from build123d import *

# Parameters (mm, degrees)
SKETCH1_W           = 21.3
SKETCH1_H           = 15.3
BOSS_EXTRUDE1_DEPTH = 1.7
BOSS_EXTRUDE2_START = 1.7
SKETCH1_3_W         = 3
SKETCH1_3_H         = 2.5
BOSS_EXTRUDE2_DEPTH = 0.9
SKETCH1_4_R         = 0.5
SKETCH1_4_R_2       = 1.5
CUT_EXTRUDE1_DEPTH  = 14.368058947


with BuildPart() as part:
    # Sketch1 → Boss-Extrude1 (new body)
    with BuildSketch(Plane.XY):
        Rectangle(SKETCH1_W, SKETCH1_H)
    extrude(amount=BOSS_EXTRUDE1_DEPTH)

    # Sketch1<3> → Boss-Extrude2 (add)
    with BuildSketch(Plane.XY.offset(BOSS_EXTRUDE2_START)):
        with Locations((0, 2.4)):
            Rectangle(SKETCH1_3_W, SKETCH1_3_H)
    extrude(amount=BOSS_EXTRUDE2_DEPTH)

    # Sketch1<4> → Cut-Extrude1 (cut, through all)
    with BuildSketch(Plane.XY):
        with Locations(Location((3.857142857, -6.4, 0), (0, 0, 180))):
            Circle(SKETCH1_4_R)
        with Locations(Location((-8.65, 5.65, 0), (0, 0, 180))):
            Circle(SKETCH1_4_R_2)
        with Locations(Location((8.65, 5.65, 0), (0, 0, 180))):
            Circle(SKETCH1_4_R_2)
        with Locations(Location((-9, -6.4, 0), (0, 0, 180))):
            Circle(SKETCH1_4_R)
        with Locations(Location((-6.428571429, -6.4, 0), (0, 0, 180))):
            Circle(SKETCH1_4_R)
        with Locations(Location((-3.857142857, -6.4, 0), (0, 0, 180))):
            Circle(SKETCH1_4_R)
        with Locations(Location((-1.285714286, -6.4, 0), (0, 0, 180))):
            Circle(SKETCH1_4_R)
        with Locations(Location((1.285714286, -6.4, 0), (0, 0, 180))):
            Circle(SKETCH1_4_R)
        with Locations(Location((6.428571429, -6.4, 0), (0, 0, 180))):
            Circle(SKETCH1_4_R)
        with Locations(Location((9, -6.4, 0), (0, 0, 180))):
            Circle(SKETCH1_4_R)
    extrude(amount=CUT_EXTRUDE1_DEPTH, mode=Mode.SUBTRACT)


solid = part.part
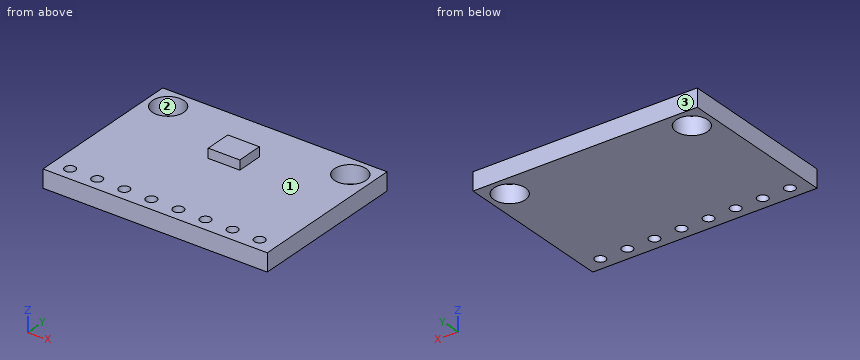
The listing builds one solid part. Answer for the finished solid, in the listing's coordinates (mm). Face numbers are marked on the shaded views. Give positions to 0.01 mm unless a question says otherwise; leave off trailing zeros. Write each loop counter-clockwise with the first axis right and the second up, starting at its lowest first coordinate (ties: lowest second). Pieces come first, ordered by that corner, then holes. Notation, with made-up numbers: (83.25, 25) -> (91.25, 25) arc R11 cw to (91.25, 37) -> close; hole circle Ø8 at (-11, 7.5). An arc over 180 degrees is marked (long way). Use a Markdown table: item, result.
(1) Section B-B, the plane x = -7.75 is taken. Determine the outline of the cut face in (y, z), then the cut area to 3 significant figures.
Return value:
| item | result |
|---|---|
| outline | (-7.65, 0) -> (4.45, 0) -> (4.45, 1.7) -> (-7.65, 1.7) -> close; (6.85, 0) -> (7.65, 0) -> (7.65, 1.7) -> (6.85, 1.7) -> close |
| area | 21.9 mm2 |
(2) Find the intervals of material crossed by probe 1 along X at (y, z) = (5.65, 1.3); probe 2 along Y at (x, z) = (8.65, 0.5); probe 3 along Z at (x, y) = (3.75, -3), in increasing order. Write a range as from..to.
Return value:
| item | result |
|---|---|
| probe 1 | -10.65..-10.15, -7.15..7.15, 10.15..10.65 |
| probe 2 | -7.65..-6.76, -6.04..4.15, 7.15..7.65 |
| probe 3 | 0..1.7 |
(3) Section C-C, the plane y = 5.65 is taken. Determine the outline of the cut face in (x, z), then the cut area to 3 significant figures.
Return value:
| item | result |
|---|---|
| outline | (-10.65, 0) -> (-10.15, 0) -> (-10.15, 1.7) -> (-10.65, 1.7) -> close; (-7.15, 0) -> (7.15, 0) -> (7.15, 1.7) -> (-7.15, 1.7) -> close; (10.15, 0) -> (10.65, 0) -> (10.65, 1.7) -> (10.15, 1.7) -> close |
| area | 26.0 mm2 |
(4) Section A-A, the plane z = 1.45 is taken. Give the number of separate pieces and of enclosed holes in the cut face, then the cut area to 3 significant figures.
Return value:
| item | result |
|---|---|
| separate pieces | 1 |
| enclosed holes | 10 |
| area | 305 mm2 |
(5) Flat-ended cylindrical pins translate along their axes: P1, Ø1.8, axis at x = -8.65, y = 5.65, coming from the +Z side; P2, Ø0.7, axis at x = -0.5, z = 2.5, coming from the -Y side; P3, Ø1, axis at x = 0, z = 2, coming from the +Y side; P4, Ø0.7, axis at y = 2, z = 2.5, coming from the +X side. Find the tip coordinate at first contact, or state that the pin passes through.
Return value:
| item | result |
|---|---|
| P1 | through |
| P2 | y = 1.15 |
| P3 | y = 7.65 |
| P4 | x = 1.5 |
(6) Section D-D, the plane x = 9 is taken. Determine the outline of the cut face in (y, z), then the cut area to 3 significant figures.
Return value:
| item | result |
|---|---|
| outline | (-7.65, 0) -> (-6.9, 0) -> (-6.9, 1.7) -> (-7.65, 1.7) -> close; (-5.9, 0) -> (4.19, 0) -> (4.19, 1.7) -> (-5.9, 1.7) -> close; (7.11, 0) -> (7.65, 0) -> (7.65, 1.7) -> (7.11, 1.7) -> close |
| area | 19.4 mm2 |
(7) Determine the mould class of the marked faces 1, 2 and 3 for opening direction Y: released by +Y, released by -Y, zero draft, split by the parting line, or undercut.
Return value:
| item | result |
|---|---|
| face 1 | zero draft |
| face 2 | undercut |
| face 3 | released by +Y |
